```python
from build123d import *

# Parameters (mm, degrees)
SKETCH003_R      = 162.0844056183
PAD002_DEPTH     = 18
SKETCH009_W      = 95
SKETCH009_H      = 95
POCKET002_DEPTH  = 1
HOLE_D           = 5
HOLE_DEPTH       = 10
HOLE_CBORE_D     = 8
HOLE_CBORE_DEPTH = 1
SKETCH011_R      = 5
POCKET003_DEPTH  = 18.001


with BuildPart() as part:
    # Sketch003 → Pad002 (new body)
    with BuildSketch(Plane.XY):
        Circle(SKETCH003_R)
    extrude(amount=PAD002_DEPTH)

    # Sketch009 (on Face3 of Pad002) → Pocket002 (cut)
    with BuildSketch(Plane.XY.offset(18)):
        Rectangle(SKETCH009_W, SKETCH009_H)
    extrude(amount=-POCKET002_DEPTH, mode=Mode.SUBTRACT)

    # Hole
    with Locations(Plane.XY.offset(17)):
        with Locations((-41.5, 41.5), (41.5, 41.5), (-41.5, -41.5), (41.5, -41.5)):
            CounterBoreHole(HOLE_D / 2, HOLE_CBORE_D / 2, HOLE_CBORE_DEPTH, depth=HOLE_DEPTH)

    # Sketch011 (on Face3 of Hole) → Pocket003 (cut, through all)
    with BuildSketch(Plane.XY.offset(18)):
        with Locations((-58.6898628385, 0)):
            Circle(SKETCH011_R)
        with Locations((0, 58.6898628385)):
            Circle(SKETCH011_R)
        with Locations((58.6898628385, 0)):
            Circle(SKETCH011_R)
        with Locations((0, -58.6898628385)):
            Circle(SKETCH011_R)
    extrude(amount=-POCKET003_DEPTH, mode=Mode.SUBTRACT)


with BuildPart() as part_1:
    # Clone004 placement: moved
    add(part.part.moved(Location((0, 0, -24))))


solid = part_1.part
```
The model under review builds one solid part; all positions refer to its coordinate system, in mm. A direction names the side the tool comes from. Round coordinates to 2 decimals unless told otherwise and drop trailing zeros. Order: outer loops, then holes, each group sorted by start corner. A loop starts at its lowest first (then second) coordinate and runs counter-clockwise, first axis right, second up.
Item 1: Add section C-C, the plane z = -11.5. Count the separate pieces of the cut face and the enclosed holes in it, and give its area (3 significant figures).
Working result:
separate pieces: 1
enclosed holes: 8
area: 82,100 mm2
Item 2: To check wall thickness, follow probe 1 along Y at (x, z) = (41.5, -13.25); probe 2 along Y at (x, z) = (-41.5, -7.15); probe 3 along X at (y, z) = (1.5, -22.25). State the ranges of each line that lie inside material, in increasing order.
Working result:
probe 1: y = -156.68 to -44, -39 to 39, 44 to 156.68
probe 2: y = -156.68 to -45.5, -37.5 to 37.5, 45.5 to 156.68
probe 3: x = -162.08 to -63.46, -53.92 to 53.92, 63.46 to 162.08
Item 3: Add section A-A, the plane x = 0. State the section outline as (y, z) points, and give its area (3 significant figures).
Working result:
outline: (-162.08, -24) - (-63.69, -24) - (-63.69, -6) - (-162.08, -6) - close; (-53.69, -24) - (53.69, -24) - (53.69, -6) - (47.5, -6) - (47.5, -7) - (-47.5, -7) - (-47.5, -6) - (-53.69, -6) - close; (63.69, -24) - (162.08, -24) - (162.08, -6) - (63.69, -6) - close
area: 5,380 mm2
Item 4: Draft analysis for pull direction X (two halves, no side actions). For faces 1 (the cylindrical face through (-128.62, -98.63, -15.13)), 2 (the cylindrical face through (-0.651, -53.732, -14.874)), 3 (the flat face through (-2, 2, -24)), state which applies: released by +X, released by -X, zero draft, split by the parting line, or undercut.
Working result:
face 1: split by the parting line
face 2: undercut
face 3: zero draft
Item 5: For pin 1 (6 mm diameter, centred on x = 101, z = -11, fed in from -Y); pin 2 (10 mm diameter, centred on x = 86, z = -13, fed in from +Y); pin 3 (1.5 mm diameter, centred on x = 41, y = 41.5, fed in from +Z); pin 4 (13 mm diameter, centred on x = 58.69, y = 0, fed in from -Z), all flat-tipped, find the tip position at first contact; note any pin that passes through.
Working result:
pin 1: stops at y = -129.1
pin 2: stops at y = 140.39
pin 3: stops at z = -17
pin 4: stops at z = -24
Item 6: Add section D-D, the plane x = 94. State the section outline as (y, z) points.
Working result:
outline: (-132.04, -24) - (132.04, -24) - (132.04, -6) - (-132.04, -6) - close
Item 7: Machinability: for faces 4 (the cylindrical face through (38.55, 44.2, -7.49)), 5 (the cylindrical face through (53.695, 0.22, -14.874)), which of the approach directions +Z, -Z, +X, -X, +Y, -Y give a long, thin tool a straight path to every point of the face, cutting with its end or side? Answer none if there is none.
Working result:
face 4: +Z
face 5: +Z, -Z
